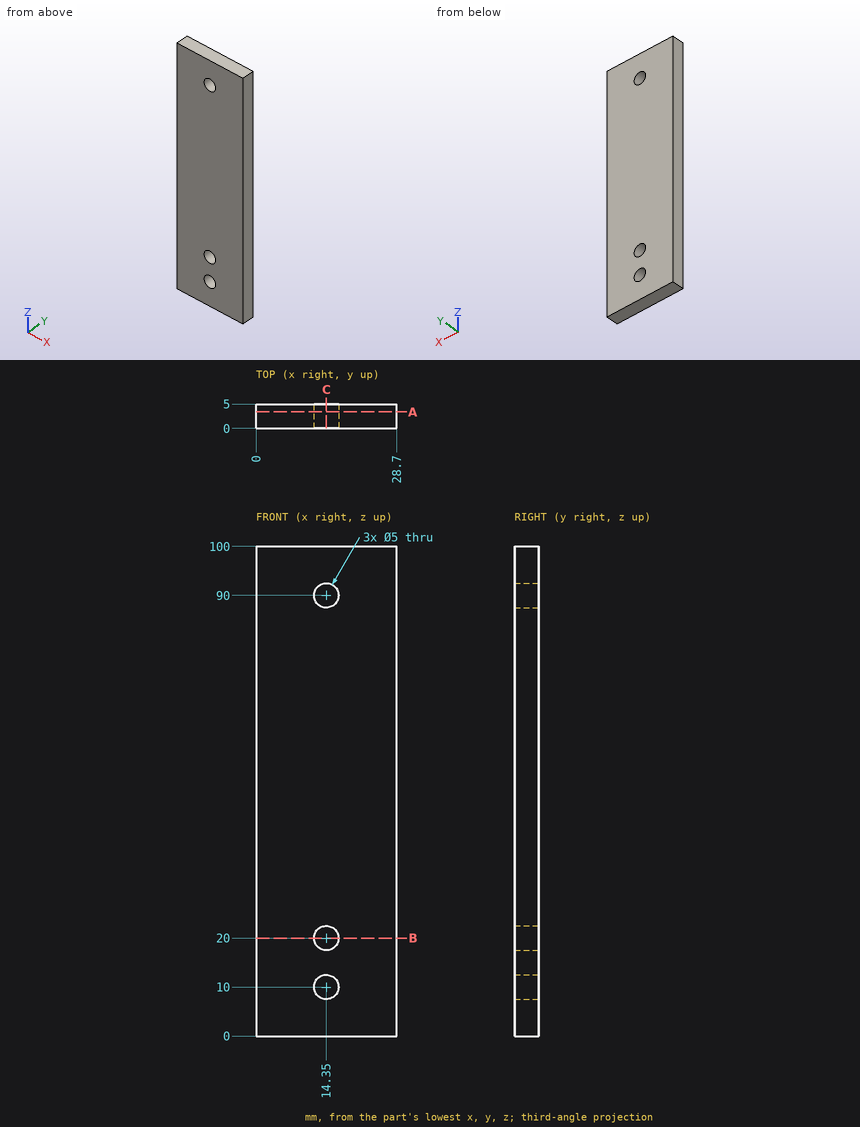
Design review of the part shown in the three views and the two pictorial views. Dimensions are in mm from the part's minimum x, y and z. Give positions to 0.01 mm unless a question says otherwise; leave off trailing zeros. Write each loop counter-clockwise with the first axis right and the second up, starting at its lowest first coordinate (ties: lowest second). Pieces come first, ordered by that corner, then holes.
(1) Add section B-B (z = 20). Give the boundary of the cut face in (x, y).
Checked values:
outline: (0, 0) - (11.85, 0) - (11.85, 5) - (0, 5) - close; (16.85, 0) - (28.7, 0) - (28.7, 5) - (16.85, 5) - close
(2) Add section C-C (x = 14.35). Give the boundary of the cut face in (y, z), and give its area (3 significant figures).
Checked values:
outline: (0, 0) - (5, 0) - (5, 7.5) - (0, 7.5) - close; (0, 12.5) - (5, 12.5) - (5, 17.5) - (0, 17.5) - close; (0, 22.5) - (5, 22.5) - (5, 87.5) - (0, 87.5) - close; (0, 92.5) - (5, 92.5) - (5, 100) - (0, 100) - close
area: 425 mm2
(3) Wall thickness on line 1 along Z through (x, y) = (14.35, 4); line 2 along X through (y, z) = (1.1, 10); line 3 along Z through (x, y) = (15, 2.15): over which ranges is each line inside the solid? List them lowest first.
Checked values:
line 1: z = 0 to 7.5, 12.5 to 17.5, 22.5 to 87.5, 92.5 to 100
line 2: x = 0 to 11.85, 16.85 to 28.7
line 3: z = 0 to 7.59, 12.41 to 17.59, 22.41 to 87.59, 92.41 to 100
(4) Add section A-A (y = 3.4). Give the boundary of the cut face in (x, z).
Checked values:
outline: (0, 0) - (28.7, 0) - (28.7, 100) - (0, 100) - close; hole circle Ø5 at (14.35, 10); hole circle Ø5 at (14.35, 20); hole circle Ø5 at (14.35, 90)
(5) Clearance check with a flat-ended pin moving along its axis: pin 1 Ø4.5 at (x, z) = (14.35, 90) entering from -Y. State where the tip first meets the part, or that it passes through.
Checked values:
pin 1: passes through
